Geometry: final body of the model. Coordinates: model frame, mm. Face numbers are marked on the shaded views. A direction names the side the tool comes from. Round coordinates to 2 decimals unless told otherwise and drop trailing zeros. Write each loop counter-clockwise with the first axis right and the second up, starting at its lowest first coordinate (ties: lowest second). Pieces come first, ordered by that corner, then holes. Notation, with made-up numbers: M -12.5,0 L 13.5,0 A10 ccw 13.5,12 Z; hole C 65.25,-11 d5. An arc over 180 degrees is marked long. Use one line per item in the form item = value. Start each with the question number.
Item 1: Section query C-C (x = 15.25). Return loops of the section in (y, z) (3 decimals), and give its area (3 significant figures).
Item 2: Section query B-B (z = 6). Return loops of the section in (x, y) (3 decimals).
Item 3: Pull-direction query (Y, two-part tool) for the marked faces 4, 5, 6 and 7; classes: pulls with the +Y half, pulls with the -Y half, needs draft (parallel to the pull), parting line crosses it, or undercut.
Item 4: Section query D-D (y = 6.5). Return loops of the section in (x, z), and give its area (3 significant figures).
Item 5: Ray query, probe 1 along X at (y, z) = (-1, 5) (3 decimals); probe 2 along X at (y, z) = (2.5, 5); probe 3 along X at (y, z) = (-0.5, 28.5) (3 decimals). Return the intervals inside material, ascending.
Item 6: Section query A-A (y = -1.5). Return loops of the section in (x, z) (3 decimals), and give its area (3 significant figures).
Item 7: Pin query (flat end, axial travel): pin 1 Ø1.4 at (y, z) = (-1.5, 3.5) entering from -X; pin 2 Ø9 at (x, z) = (14.5, 9.5) entering from -Y; pin 3 Ø10 at (y, z) = (4.5, 22) entering from -X; pin 4 Ø1.9 at (y, z) = (-2.5, 27.5) entering from +X. Return the tip coordinate at first contact, or that it passes through.
Item 8: Reachability of the marked faces 1, 2 and 3 from +Z, -Z, +X, -X, +Y, -Y: full face, straight path, thin tool, end or side. Return the list, or none.
from build123d import *

# Parameters (mm, degrees)
BOSS_EXTRUDE1_DEPTH = 31.75
SKETCH2_W           = 16.51
SKETCH2_H           = 2.54
CUT_EXTRUDE1_DEPTH  = 31.75
SKETCH3_W           = 16.51
SKETCH3_H           = 2.54
CUT_EXTRUDE2_DEPTH  = 31.75


with BuildPart() as part:
    # Sketch1 → Boss-Extrude1 (new body)
    with BuildSketch(Plane.XY):
        Polygon((2.413, -2.54), (2.413, -0.750440267), (3.048, -0.750440267), (3.048, -3.175), (0, -3.175), (0, 0.635), (18.127436567, 0.635), (13.348744151, 13.135564727), (0, 0.889), (-2.575678152, 3.696486787), (-0.329688722, 5.757029308), (1.387430046, 3.88537145), (0.919515581, 3.456091758), (-0.368323494, 4.859835152), (-1.678483995, 3.657852015), (0.038634773, 1.786194156), (13.608154244, 14.235305222), (19.05, 0), (0.635, 0), (0.635, -2.54), align=None)
    extrude(amount=BOSS_EXTRUDE1_DEPTH)

    # Sketch2 → Cut-Extrude1 (cut)
    with BuildSketch(Plane(origin=(0.442854564, 0.406288938, 0), x_dir=(0, 0, 1), z_dir=(-0.7368731724730907, -0.676031010893319, 0))):
        with Locations((15.875, 3.19508025)):
            Rectangle(SKETCH2_W, SKETCH2_H)
    extrude(amount=-CUT_EXTRUDE1_DEPTH, mode=Mode.SUBTRACT)

    # Sketch3 → Cut-Extrude2 (cut)
    with BuildSketch(Plane.ZY):
        with Locations((15.875, -1.905)):
            Rectangle(SKETCH3_W, SKETCH3_H)
    extrude(amount=-CUT_EXTRUDE2_DEPTH, mode=Mode.SUBTRACT)


solid = part.part
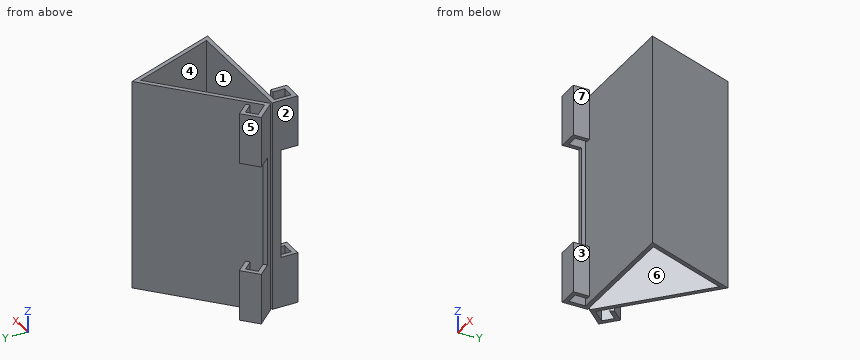
Working result:
q1.outline = M 0,0 L 0.635,0 L 0.635,31.75 L 0,31.75 Z; M 8.162,0 L 9.94,0 L 9.94,31.75 L 8.162,31.75 Z
q1.area = 76.6 mm²
q2.outline = M -2.576,3.696 L 0,0.889 L 13.349,13.136 L 18.127,0.635 L 0,0.635 L 0,-3.175 L 3.048,-3.175 L 3.048,-0.75 L 2.413,-0.75 L 2.413,-2.54 L 0.635,-2.54 L 0.635,0 L 19.05,0 L 13.608,14.235 L 0.039,1.786 L -1.678,3.658 L -0.368,4.86 L 0.92,3.456 L 1.387,3.885 L -0.33,5.757 Z
q3.face_4 = undercut
q3.face_5 = pulls with the +Y half
q3.face_6 = undercut
q3.face_7 = needs draft
q4.outline = M 5.18,0 L 6.12,0 L 6.12,31.75 L 5.18,31.75 Z; M 15.89,0 L 16.57,0 L 16.57,31.75 L 15.89,31.75 Z
q4.area = 51.4 mm²
q5.probe_1 = 0 to 0.635, 2.413 to 3.048
q5.probe_2 = -1.48 to -0.62, 0.82 to 1.76, 17.41 to 18.09
q5.probe_3 = 0 to 0.635
q6.outline = M 0,0 L 0.635,0 L 0.635,7.62 L 0,7.62 Z; M 0,24.13 L 0.635,24.13 L 0.635,31.75 L 0,31.75 Z; M 2.413,0 L 3.048,0 L 3.048,7.62 L 2.413,7.62 Z; M 2.413,24.13 L 3.048,24.13 L 3.048,31.75 L 2.413,31.75 Z
q6.area = 19.4 mm²
q7.pin_1 = 0
q7.pin_2 = 0
q7.pin_3 = -2.58
q7.pin_4 = 3.05
q8.face_1 = +Z, -Z, -X
q8.face_2 = +Z, -Z, -X, -Y
q8.face_3 = +Z, -Z, +X, -Y
